from build123d import *

# Parameters (mm, degrees)
F1_DEPTH      = 914.4
F4_DEPTH      = 50.8
F4_DEPTH_BACK = 25.4
F5_DEPTH      = 50.8


with BuildPart() as f1:
    # F0 (on Top) → F1 (new body)
    with BuildSketch(Plane.XY):
        Polygon((10.0081935422, 9.9204859395), (10.0081935422, 30.1515859395), (8.4206935422, 30.1515859395), (8.4206935422, 9.4563106097), (1.6738185422, 2.6999106097), (1.6738185422, 30.1515859395), (0.0863185422, 30.1515859395), (0.0863185422, -0.0109140605), (30.2488185422, -0.0109140605), (30.2488185422, 1.5765859395), (2.7955595779, 1.5765859395), (9.5424345779, 8.3329859395), (30.2488185422, 8.3329859395), (30.2488185422, 9.9204859395), align=None)
    extrude(amount=F1_DEPTH)

    # F2 (on Front) → F4 (cut, two sides)
    with BuildSketch(Plane.XZ) as f4_sk:
        Polygon((30.48, 30.48), (0, 0), (30.48, 0), align=None)
    extrude(amount=-F4_DEPTH, mode=Mode.SUBTRACT)
    extrude(f4_sk.sketch, amount=F4_DEPTH_BACK, mode=Mode.SUBTRACT)

    # F3 (on Right) → F5 (cut)
    with BuildSketch(Plane.YZ):
        Polygon((30.1625, 30.1625), (0, 0), (30.1625, 0), align=None)
    extrude(amount=F5_DEPTH, mode=Mode.SUBTRACT)


solid = f1.part
Verification items for the finished model (mm, model axes). A direction names the side the tool comes from. Give positions to 0.01 mm unless a question says otherwise; leave off trailing zeros. Order: outer loops, then holes, each group sorted by start corner. A loop starts at its lowest first (then second) coordinate and runs counter-clockwise, first axis right, second up. Notation, with made-up numbers: M 55.25,26 L 82.25,26 A15 cw 82.25,51 Z; hole C -9,36 d4. An arc over 180 degrees is marked long. Answer as a JSON object with one key per item and string values. Group by question number.
1) Cross-section at C-C (z = 631). Enter the section's corners in (x, y).
2) Cross-section at A-A (y = 21). Enter the section's corners in (x, z).
3) Mould release check, pull along X, two halves, no side actions. Record for faces 5 (the face through (20, 9.92, 456)), 6 (the face through (1.674, 16, 452)), 7 (the face through (0.086, 15, 451)): released by +X, released by -X, zero draft, split by the parting line, or undercut.
4) Scan lines: line 1 along Y through (x, z) = (25, 255); line 2 along X through (y, z) = (17, 305); line 3 along X through (y, z) = (3, 181.5). Record each from-to range of solid material in increasing order. Write a range as [from, to].
5) Access from +Z, -Z, +X, -X, +Y, -Y to the whole of each face (thin tool, end or side, straight path). Record for faces 1 (the face through (8.421, 20, 456)), 2 (the face through (20, 8.333, 456)), 3 (the face through (10.008, 20, 456)), 4 (the face through (15, -0.011, 451)).
6) Depth check by flat-ended pin: pin 1 Ø16 at (y, z) = (21, 603.5) entering from +X; pin 2 Ø2 at (x, z) = (4, 149.5) entering from +Y; pin 3 Ø10 at (x, z) = (20, 477.5) entering from +Y. Enter the tip coordinate at first touch or a pass-through.
7) Cross-section at B-B (x = 23). Enter the section's corners in (y, z).
Result sheet:
{
 "1": {"outline": "M 0.09,-0.01 L 30.25,-0.01 L 30.25,1.58 L 2.8,1.58 L 9.54,8.33 L 30.25,8.33 L 30.25,9.92 L 10.01,9.92 L 10.01,30.15 L 8.42,30.15 L 8.42,9.46 L 1.67,2.7 L 1.67,30.15 L 0.09,30.15 Z"},
 "2": {"outline": "M 0.09,21 L 1.67,21 L 1.67,914.4 L 0.09,914.4 Z; M 8.42,21 L 10.01,21 L 10.01,914.4 L 8.42,914.4 Z"},
 "3": {"face 5": "zero draft", "face 6": "undercut", "face 7": "released by -X"},
 "4": {"line 1": "y = [-0.01, 1.58], [8.33, 9.92]", "line 2": "x = [0.09, 1.67], [8.42, 10.01]", "line 3": "x = [0.09, 1.67], [1.97, 4.22]"},
 "5": {"face 1": "+Z, -Z, +Y", "face 2": "+Z, -Z, +X", "face 3": "+Z, -Z, +X, +Y", "face 4": "+Z, -Z, +X, -X, -Y"},
 "6": {"pin 1": "stops at x = 10.01", "pin 2": "stops at y = 6.03", "pin 3": "stops at y = 9.92"},
 "7": {"outline": "M -0.01,23 L 1.58,23 L 1.58,914.4 L -0.01,914.4 Z; M 8.33,23 L 9.92,23 L 9.92,914.4 L 8.33,914.4 Z"}
}
